Autodesk Inventor part; units mm, degrees
ref_plane "YZ Plane" through (0, 0, 0) normal (1, 0, 0) x (0, 1, 0)
ref_plane "XZ Plane" through (0, 0, 0) normal (0, 1, 0) x (-1, 0, 0)
ref_plane "XY Plane" through (0, 0, 0) normal (0, 0, 1) x (1, 0, 0)
sketch "Sketch1" plane through (0, 0, 0) normal (0, 1, 0) x (-1, 0, 0)
  line L0 (555, 500) -> (-555, 500)
  line L1 (-555, 500) -> (-555, -500)
  line L2 (-555, -500) -> (555, -500)
  line L3 (555, -500) -> (555, 500)
  line L4 (555, 500) -> (-555, -500) construction
  line L5 (-555, 500) -> (555, -500) construction
  line L6 (235, 50) -> (505, 50)
  line L7 (505, 50) -> (505, 450)
  line L8 (505, 450) -> (235, 450)
  line L9 (235, 450) -> (235, 50)
  line L10 (-135, 50) -> (135, 50)
  line L11 (135, 50) -> (135, 450)
  line L12 (135, 450) -> (-135, 450)
  line L13 (-135, 450) -> (-135, 50)
  line L14 (-505, 50) -> (-235, 50)
  line L15 (-235, 50) -> (-235, 450)
  line L16 (-235, 450) -> (-505, 450)
  line L17 (-505, 450) -> (-505, 50)
  line L18 (235, -450) -> (505, -450)
  line L19 (505, -450) -> (505, -50)
  line L20 (505, -50) -> (235, -50)
  line L21 (235, -50) -> (235, -450)
  line L22 (-135, -450) -> (135, -450)
  line L23 (135, -450) -> (135, -50)
  line L24 (135, -50) -> (-135, -50)
  line L25 (-135, -50) -> (-135, -450)
  line L26 (-505, -450) -> (-235, -450)
  line L27 (-235, -450) -> (-235, -50)
  line L28 (-235, -50) -> (-505, -50)
  line L29 (-505, -50) -> (-505, -450)
  line L30 (-555, 500) -> (-1155, 500)
  line L31 (-1155, 500) -> (-1155, -500)
  line L32 (-1155, -500) -> (-555, -500)
  line L33 (-555, -500) -> (-555, 500)
  line L34 (-555, 500) -> (-1155, 500)
  line L35 (-1155, 500) -> (-1155, 450)
  line L36 (-1155, 450) -> (-555, 450)
  line L37 (-555, 450) -> (-555, 500)
  line L38 (-555, -500) -> (-1155, -500)
  line L39 (-1155, -500) -> (-1155, -450)
  line L40 (-1155, -450) -> (-555, -450)
  line L41 (-555, -450) -> (-555, -500)
  line L42 (-1155, -500) -> (555, -500)
  line L43 (555, -500) -> (555, -550)
  line L44 (555, -550) -> (-1155, -550)
  line L45 (-1155, -550) -> (-1155, -500)
  line L46 (-1155, 500) -> (555, 500)
  line L47 (555, 500) -> (555, 550)
  line L48 (555, 550) -> (-1155, 550)
  line L49 (-1155, 550) -> (-1155, 500)
  line L50 (-555, 450) -> (-1155, 450)
  line L51 (-1155, 450) -> (-1155, -150)
  line L52 (-1155, -150) -> (-555, -150)
  line L53 (-555, -150) -> (-555, 450)
  point P0 (0, 0)
  point P1 (555, -525)
  dimension "d0" = 1000
  dimension "d1" = 1110
  dimension "d2" = 400
  dimension "d3" = 270
  dimension "d4" = 50
  dimension "d5" = 50
  dimension "d8" = 370
  dimension "d11" = 500
  dimension "d14" = 600
  dimension "d15" = 50
  dimension "d16" = 50
  dimension "d17" = 50
  dimension "d18" = 50
  dimension "d19" = 600
  dimension "d26" = 0
  dimension "d27" = 0
extrude "Extrusion1" add sketch "Sketch1" along normal blind 25 contours L3 L2 L1 L0 | L0 L30 L49 L48 L47 | L1 L36 L31 L30 | L43 L44 L45 L32 L2 | L32 L31 L40 L1 | L1 L40 L31 L52 | L9 L8 L7 L6 | L13 L12 L11 L10 | L17 L16 L15 L14 | L21 L20 L19 L18 | L25 L24 L23 L22 | L29 L28 L27 L26
fillet "Fillet1" radius 20 4 edges at (555, 12.5, -150) (555, 12.5, 450) (1155, 12.5, 450) (1155, 12.5, -150)
chamfer "Chamfer1" distance 2 angle 45 20 edges at (855, 0, -150) (1149.1421, 0, -155.8579) (1155, 0, -335) (555, 0, 150) (855, 0, 450) (1149.1421, 0, 455.8579) (1155, 0, 485) (300, 0, 550) (-555, 0, 0) (300, 0, -550) (1155, 25, -335) (1149.1421, 25, -155.8579) (855, 25, -150) (555, 25, 150) (855, 25, 450) (1149.1421, 25, 455.8579) (1155, 25, 485) (300, 25, 550) (-555, 25, 0) (300, 25, -550)
equation "\"d0\" = Grundplatte_Width"
equation "\"d1\" = Grundplatte_Hight"
equation "\"d2\" = Palette_Width"
equation "\"d3\" = Palette_Hight"
equation "\"d4\" = Palette_Padding_Outer"
equation "\"d5\" = Palette_Padding_Outer"
equation "\"d8\" = Palette_Padding_Inner_X"
equation "\"d11\" = Palette_Padding_Inner_Y"
equation "\"d15\" = Palette_Padding_Outer"
equation "\"d16\" = Palette_Padding_Outer"
equation "\"d17\" = Palette_Padding_Outer"
equation "\"d18\" = Palette_Padding_Outer"
equation "\"Palette_Width\" = 400"
equation "\"Palette_Hight\" = 270"
equation "\"Palette_Padding_Outer\" = 0.5 * Palette_Padding"
equation "\"Palette_Padding_Inner_X\" = Palette_Hight + Palette_Padding"
equation "\"Palette_Padding_Inner_Y\" = Palette_Width + Palette_Padding"
properties part number "Grundplatte"
Model file for the job. Use its own axes, mm. Give positions to 0.01 mm unless a question says otherwise; leave off trailing zeros. Loops run counter-clockwise (first coordinate to the right, second up) from the corner with the lowest first, then second, coordinate; pieces in that order, holes last. Notation, with made-up numbers: (76, -14.75) - (100, -14.75) arc R20 ccw to (100, 8.25) - close; hole circle Ø5 at (48, -36.5). An arc over 180 degrees is marked (long way). Use one line per item in the form item = value.
(1) Drill centre lines: L1, parallel to Z at x = 576.5, y = 15.75; L2, parallel to X at y = 11, z = 47.5; L3, parallel to X at y = 4.75, z = 433.5. Where is each one in solid material? Low to high.
Determined:
L1 = -550 to -150, 450 to 550
L2 = -555 to 555
L3 = -555 to 555.31
(2) Cut at A-A (y = 7.75). Give the cut face in (x, z), then the cut area to 3 significant figures.
Determined:
outline = (-555, -550) - (1155, -550) - (1155, -170) arc R20 ccw to (1135, -150) - (575, -150) arc R20 cw to (555, -130) - (555, 430) arc R20 cw to (575, 450) - (1135, 450) arc R20 ccw to (1155, 470) - (1155, 550) - (-555, 550) - close
area = 1,520,000 mm^2
(3) Cut at C-C (z = 198). Give the cut face in (x, y), then the cut area to 3 significant figures.
Determined:
outline = (-555, 2) - (-553, 0) - (553, 0) - (555, 2) - (555, 23) - (553, 25) - (-553, 25) - (-555, 23) - close
area = 27,700 mm^2
(4) Cut at B-B (x = 792). Give the cut face in (y, z).
Determined:
outline = (0, -548) - (2, -550) - (23, -550) - (25, -548) - (25, -152) - (23, -150) - (2, -150) - (0, -152) - close; (0, 452) - (2, 450) - (23, 450) - (25, 452) - (25, 548) - (23, 550) - (2, 550) - (0, 548) - close
